The listing builds one solid part. Answer for the finished solid, in the listing's coordinates (mm). Face numbers are marked on the shaded views. A direction names the side the tool comes from. Give positions to 0.01 mm unless a question says otherwise; leave off trailing zeros. Write each loop counter-clockwise with the first axis right and the second up, starting at its lowest first coordinate (ties: lowest second). Pieces come first, ordered by that corner, then holes. Notation, with made-up numbers: M 50.5,19 L 57.5,19 A23 ccw 57.5,31 Z; hole C 51.5,49.25 d2. An arc over 180 degrees is marked long. Answer as a JSON object with one key per item and string values.
```python
from build123d import *

# Parameters (mm, degrees)
F0_R     = 7
F1_DEPTH = 48.5
F2_R     = 2.7
F3_DEPTH = 1.5
F4_R     = 0.75


with BuildPart() as f1:
    # F0 (on Top) → F1 (new body)
    with BuildSketch(Plane.XY):
        Circle(F0_R)
    extrude(amount=F1_DEPTH)

    # F2 (on face) → F3 (join)
    with BuildSketch(Plane.XY.offset(48.5)):
        Circle(F2_R)
    extrude(amount=F3_DEPTH)

    # F4
    f4_edges = [f1.edges().sort_by_distance(p)[0] for p in [
        (-2.7, 0, 50),
        (-7, 0, 48.5),
        (-7, 0, 0),
    ]]
    fillet(f4_edges, radius=F4_R)


solid = f1.part
```
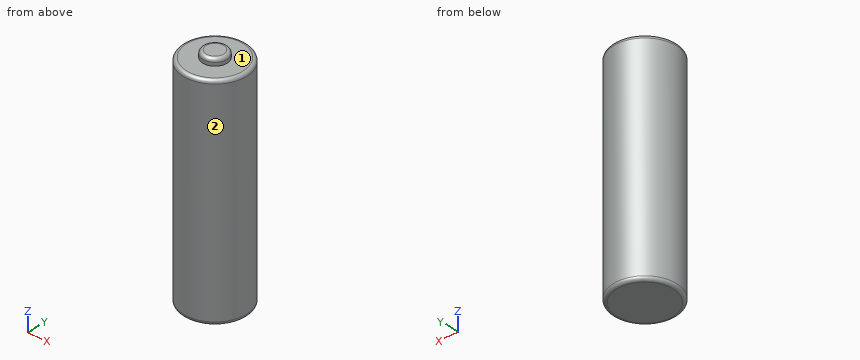
1. Consider line 1 along Z through (x, y) = (0, -3.75); line 2 along X through (y, z) = (1.25, 45.5); line 3 along X through (y, z) = (3, 31). Determine where each line is inside the solid, lowest interval first.
Verdict:
{"line 1": "z = 0 to 48.5", "line 2": "x = -6.89 to 6.89", "line 3": "x = -6.32 to 6.32"}
2. For the marked faces 1 and 2, determine the directions among +Z, -Z, +X, -X, +Y, -Y from which every point of the face is accessible in a straight line to the end or side of a thin tool.
Verdict:
{"face 1": "+Z", "face 2": "+Z, -Z"}
3. A cutting plane is placed at A-A, the plane x = 0. Give the vertices of the cut face in (y, z).
Verdict:
{"outline": "M -7,0.75 A0.75 ccw -6.25,0 L 6.25,0 A0.75 ccw 7,0.75 L 7,47.75 A0.75 ccw 6.25,48.5 L 2.7,48.5 L 2.7,49.25 A0.75 ccw 1.95,50 L -1.95,50 A0.75 ccw -2.7,49.25 L -2.7,48.5 L -6.25,48.5 A0.75 ccw -7,47.75 Z"}
4. A cutting plane is placed at C-C, the plane z = 40.5. Give the vertices of the cut face in (x, y), plus the area to 3 significant figures.
Verdict:
{"outline": "C 0,0 d14", "area": "154 mm2"}
5. Flat-ended cylindrical pins translate along their axes: pin 1 (5 mm diameter, centred on x = -3, z = 13.5, fed in from -Y); pin 2 (5 mm diameter, centred on y = 1, z = 11, fed in from -X); pin 3 (2 mm diameter, centred on x = 4, y = 1, fed in from +Z); pin 4 (1 mm diameter, centred on x = 4.5, z = 20.5, fed in from -Y). Find the tip coordinate at first contact, or state that the pin passes through.
Verdict:
{"pin 1": "stops at y = -6.98", "pin 2": "stops at x = -7", "pin 3": "stops at z = 48.5", "pin 4": "stops at y = -5.74"}
